Part print with two shaded views. Sizes in mm from the minimum x, y, z corner. Coordinates: 2 decimals unless noted, no trailing zeros. Loops run counter-clockwise (first coordinate to the right, second up) from the corner with the lowest first, then second, coordinate; pieces in that order, holes last. Notation, with made-up numbers: (88, 14) -> (107, 14) arc R15 cw to (107, 30) -> close; hole circle Ø9 at (-31, -36). An arc over 180 degrees is marked (long way). Use one line per item in the form item = value.
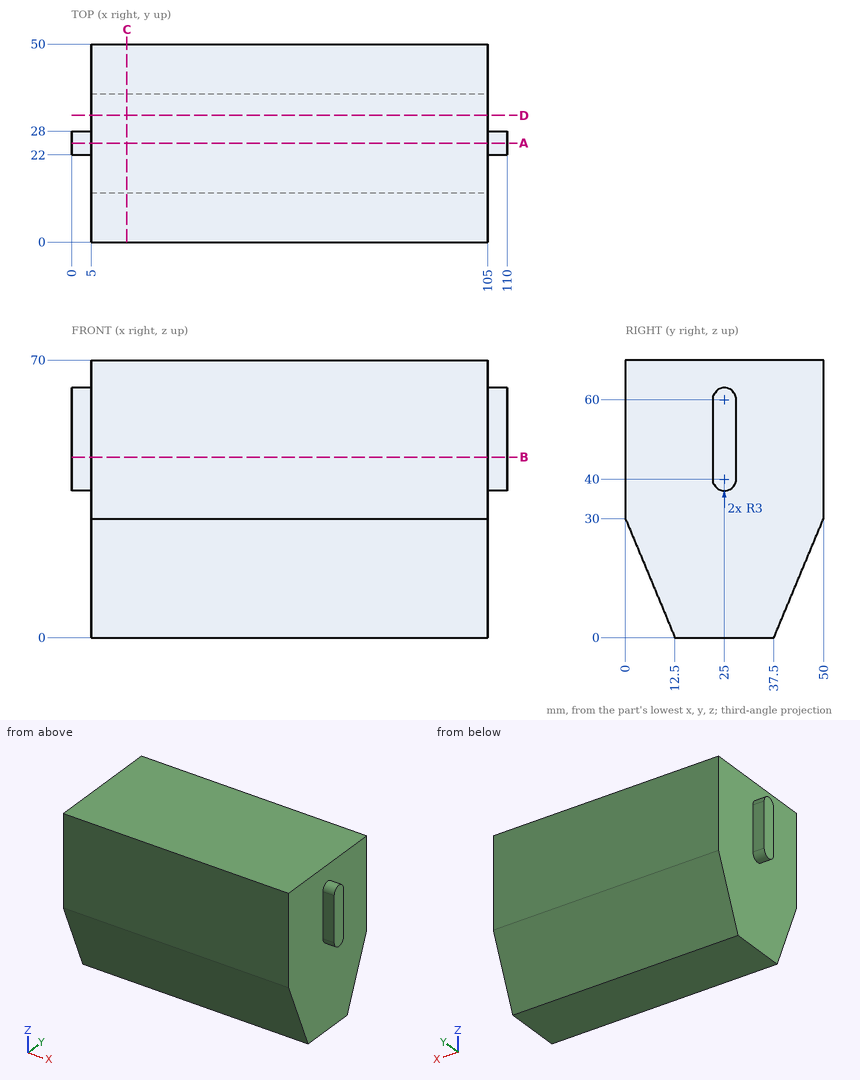
Q1. Pin check, flat tips, straight feed: pin 1 Ø4 at (x, z) = (3.5, 51) entering from +Y; pin 2 Ø1.5 at (y, z) = (42, 61) entering from -X; pin 3 Ø1.5 at (y, z) = (26.5, 27.5) entering from +X; pin 4 Ø2.5 at (x, z) = (3, 45) entering from -Y. Stop position of each tip, or through.
Result:
pin_1 = 50
pin_2 = 5
pin_3 = 105
pin_4 = 22
Q2. Band-saw the part on D-D, the plane y = 32. Write the cut outline in (x, z).
Result:
outline = (5, 0) -> (105, 0) -> (105, 70) -> (5, 70) -> close
Q3. Wall check: line 1 along X through (y, z) = (31, 45.5); line 2 along Y through (x, z) = (76.5, 25); line 3 along Y through (x, z) = (16, 11.5). Give the ranges that are in metal, low to high.
Result:
line_1 = 5 to 105
line_2 = 2.08 to 47.92
line_3 = 7.71 to 42.29
Q4. Band-saw the part on A-A, the plane y = 25. Write the cut outline in (x, z).
Result:
outline = (0, 37) -> (5, 37) -> (5, 0) -> (105, 0) -> (105, 37) -> (110, 37) -> (110, 63) -> (105, 63) -> (105, 70) -> (5, 70) -> (5, 63) -> (0, 63) -> close
Q5. Band-saw the part on B-B, the plane z = 45.5. Write the cut outline in (x, y).
Result:
outline = (0, 22) -> (5, 22) -> (5, 0) -> (105, 0) -> (105, 22) -> (110, 22) -> (110, 28) -> (105, 28) -> (105, 50) -> (5, 50) -> (5, 28) -> (0, 28) -> close
Q6. Band-saw the part on C-C, the plane x = 14. Write the cut outline in (y, z), and give its area (4 significant figures).
Result:
outline = (0, 30) -> (12.5, 0) -> (37.5, 0) -> (50, 30) -> (50, 70) -> (0, 70) -> close
area = 3,125 mm2
